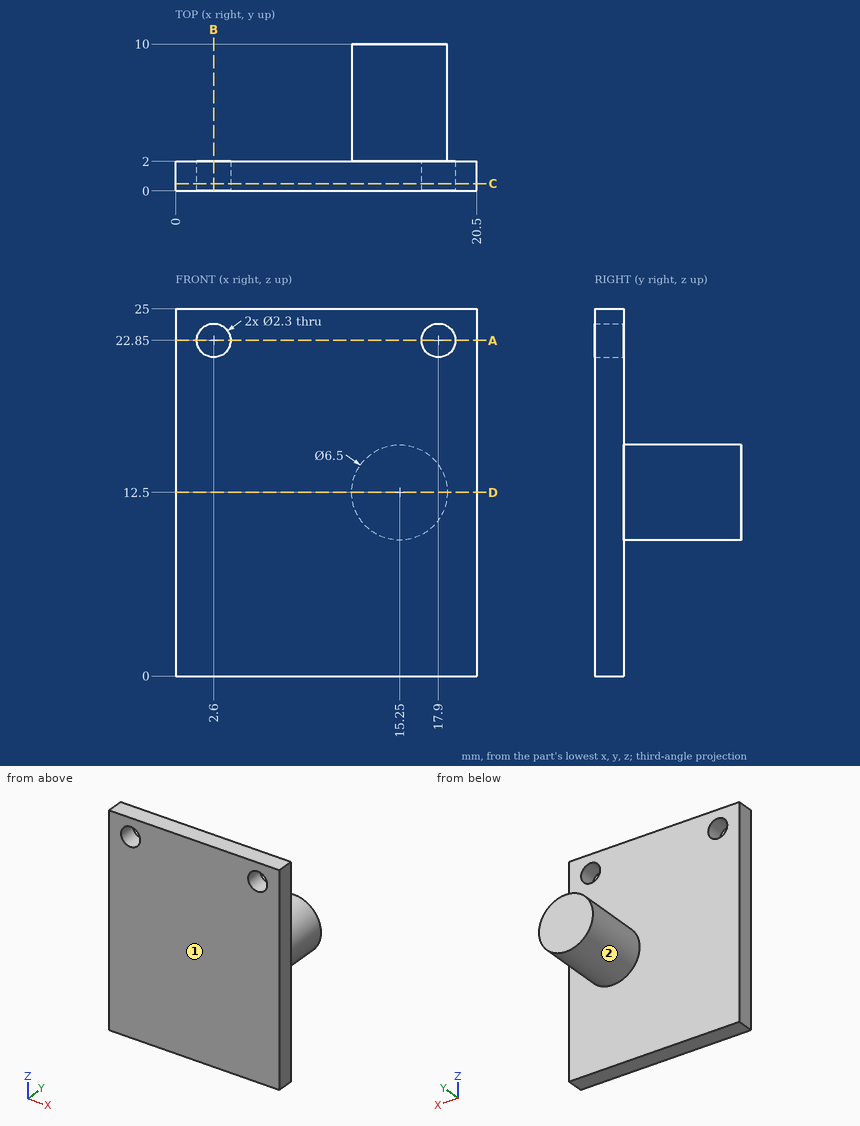
Could you check a few things on this drawing? It's one solid part, dimensions in mm from its lowest x, y, z. A direction names the side the tool comes from. Coordinates: 2 decimals unless noted, no trailing zeros. Order: outer loops, then holes, each group sorted by start corner. A loop starts at its lowest first (then second) coordinate and runs counter-clockwise, first axis right, second up. Notation, with made-up numbers: M 19.25,40.5 L 41.25,40.5 A10 cw 41.25,45.5 Z; hole C -5,26.25 d4. An arc over 180 degrees is marked long. Answer as a JSON object with one key per item and string values. Group by question number.
(1) I need wall thicknesses on probe 1 along X at (y, z) = (1.5, 22.85); probe 2 along Z at (x, y) = (17.9, 1.3); probe 3 along Y at (x, z) = (3.5, 1.5). Which ranges of each line are inside material? Lowest first, please.
(2) For pin 1 (2.5 mm diameter, centred on x = 17.9, z = 22.85, fed in from +Y); pin 2 (10 mm diameter, centred on x = 5.5, z = 7, fed in from -Y), each with a flat end and sliding along its axis, tell me the tip position at first contact or that it passes through.
(3) Which directions (+Z, -Z, +X, -X, +Y, -Y) give clear straight access to the entire face, cutting with the end or side of a thin tool? Please do the marked faces 1 and 2.
(4) Suppose I cut it at B-B, the plane x = 2.6. Please give me the cut outline in (y, z).
(5) Suppose I cut it at D-D, the plane z = 12.5. Please give me the cut outline in (x, y), then the cut area to 3 significant figures.
(6) Suppose I cut it at C-C, the plane y = 0.5. Please give me the cut outline in (x, z).
(7) Suppose I cut it at A-A, the plane z = 22.85. Please give me the cut outline in (x, y), then the cut area to 3 significant figures.
Values found:
{
 "1": {"probe 1": "x = 0 to 1.45, 3.75 to 16.75, 19.05 to 20.5", "probe 2": "z = 0 to 21.7, 24 to 25", "probe 3": "y = 0 to 2"},
 "2": {"pin 1": "stops at y = 2", "pin 2": "stops at y = 0"},
 "3": {"face 1": "+Z, -Z, +X, -X, -Y", "face 2": "+Y"},
 "4": {"outline": "M 0,0 L 2,0 L 2,21.7 L 0,21.7 Z; M 0,24 L 2,24 L 2,25 L 0,25 Z"},
 "5": {"outline": "M 0,0 L 20.5,0 L 20.5,2 L 18.5,2 L 18.5,10 L 12,10 L 12,2 L 0,2 Z", "area": "93.0 mm^2"},
 "6": {"outline": "M 0,0 L 20.5,0 L 20.5,25 L 0,25 Z; hole C 2.6,22.85 d2.3; hole C 17.9,22.85 d2.3"},
 "7": {"outline": "M 0,0 L 1.45,0 L 1.45,2 L 0,2 Z; M 3.75,0 L 16.75,0 L 16.75,2 L 3.75,2 Z; M 19.05,0 L 20.5,0 L 20.5,2 L 19.05,2 Z", "area": "31.8 mm^2"}
}
